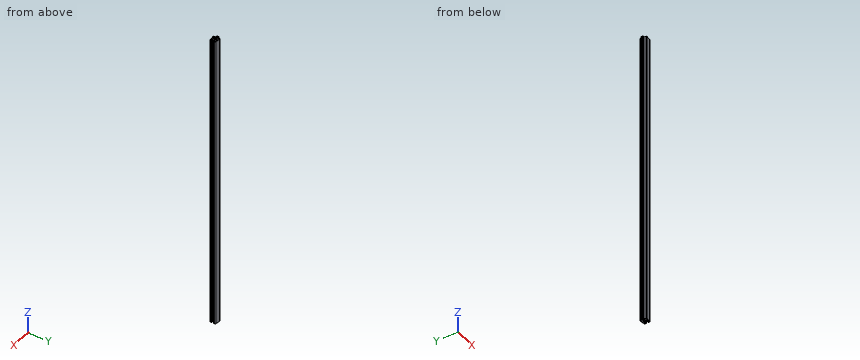
from build123d import *

# Parameters (mm, degrees)
EXTRUDE1_DEPTH = 1300


with BuildPart() as part:
    # Sketch1 → Extrude1 (new body)
    with BuildSketch(Plane.XY):
        with BuildLine():
            Line((21.490009074, 1.2), (22.34167412, 1.2))
            ThreePointArc((22.34167412, 1.2), (22.757184066, 1.325619119), (23.033504697, 1.66039604))
            ThreePointArc((23.033504697, 1.66039604), (23.959440841, 3.040559159), (25.33960396, 3.966495303))
            ThreePointArc((25.33960396, 3.966495303), (25.674380881, 4.242815934), (25.8, 4.65832588))
            Line((25.8, 4.65832588), (25.8, 5.509990926))
            ThreePointArc((25.8, 5.509990926), (25.846470105, 5.638164914), (25.964285714, 5.706776316))
            ThreePointArc((25.964285714, 5.706776316), (27, 5.8), (28.035714286, 5.706776316))
            ThreePointArc((28.035714286, 5.706776316), (28.153529895, 5.638164914), (28.2, 5.509990926))
            Line((28.2, 5.509990926), (28.2, 4.65832588))
            ThreePointArc((28.2, 4.65832588), (28.325619119, 4.242815934), (28.66039604, 3.966495303))
            ThreePointArc((28.66039604, 3.966495303), (30.040559159, 3.040559159), (30.966495303, 1.66039604))
            ThreePointArc((30.966495303, 1.66039604), (31.242815934, 1.325619119), (31.65832588, 1.2))
            Line((31.65832588, 1.2), (34.3, 1.2))
            Line((34.3, 1.2), (34.3, 5.944365081))
            ThreePointArc((34.3, 5.944365081), (34.315224093, 6.020901768), (34.358578644, 6.085786438))
            Line((34.358578644, 6.085786438), (39.053219906, 10.7804277))
            ThreePointArc((39.053219906, 10.7804277), (39.09082989, 10.804079854), (39.134973737, 10.809105395))
            Line((39.134973737, 10.809105395), (39.165647289, 10.805697223))
            ThreePointArc((39.165647289, 10.805697223), (40.117692027, 10.315253814), (40.5, 9.314871621))
            Line((40.5, 9.314871621), (40.5, 4.3))
            ThreePointArc((40.5, 4.3), (40.558578644, 4.158578644), (40.7, 4.1))
            Line((40.7, 4.1), (41.8, 4.1))
            ThreePointArc((41.8, 4.1), (41.941421356, 4.158578644), (42, 4.3))
            Line((42, 4.3), (42, 9.314871621))
            ThreePointArc((42, 9.314871621), (41.235384054, 11.315636008), (39.331294578, 12.296522825))
            Line((39.331294578, 12.296522825), (18.331294578, 14.629856158))
            ThreePointArc((18.331294578, 14.629856158), (15.999235613, 13.883589008), (15, 11.648204954))
            Line((15, 11.648204954), (15, 3.87298837))
            ThreePointArc((15, 3.87298837), (14.684748025, 3.408372219), (14.13652733, 3.529640706))
            ThreePointArc((14.13652733, 3.529640706), (13.848340865, 3.811685359), (13.538931751, 4.070271178))
            ThreePointArc((13.538931751, 4.070271178), (13.510259193, 4.105338584), (13.5, 4.149458734))
            Line((13.5, 4.149458734), (13.5, 5.04003891))
            ThreePointArc((13.5, 5.04003891), (13.470710678, 5.110749588), (13.4, 5.14003891))
            Line((13.4, 5.14003891), (10.4, 5.14003891))
            ThreePointArc((10.4, 5.14003891), (10.279875007, 5.138635031), (10.159815633, 5.134424161))
            ThreePointArc((10.159815633, 5.134424161), (8.129682846, 4.208865984), (7.3, 2.137701227))
            Line((7.3, 2.137701227), (7.3, 0.95))
            ThreePointArc((7.3, 0.95), (7.358578644, 0.808578644), (7.5, 0.75))
            Line((7.5, 0.75), (7.872649609, 0.75))
            ThreePointArc((7.872649609, 0.75), (7.986504617, 0.785570571), (8.059860749, 0.87962963))
            ThreePointArc((8.059860749, 0.87962963), (9.999819413, 2.467763258), (12.342238608, 1.574074074))
            ThreePointArc((12.342238608, 1.574074074), (12.4115514, 1.519465813), (12.497617696, 1.5))
            Line((12.497617696, 1.5), (13.5, 1.5))
            ThreePointArc((13.5, 1.5), (15, 0), (13.5, -1.5))
            Line((13.5, -1.5), (12.497617696, -1.5))
            ThreePointArc((12.497617696, -1.5), (12.4115514, -1.519465813), (12.342238608, -1.574074074))
            ThreePointArc((12.342238608, -1.574074074), (9.999819413, -2.467763258), (8.059860749, -0.87962963))
            ThreePointArc((8.059860749, -0.87962963), (7.986504617, -0.785570571), (7.872649609, -0.75))
            Line((7.872649609, -0.75), (7.5, -0.75))
            ThreePointArc((7.5, -0.75), (7.358578644, -0.808578644), (7.3, -0.95))
            Line((7.3, -0.95), (7.3, -2.137701227))
            ThreePointArc((7.3, -2.137701227), (8.129682846, -4.208865984), (10.159815633, -5.134424161))
            ThreePointArc((10.159815633, -5.134424161), (10.279875007, -5.138635031), (10.4, -5.14003891))
            Line((10.4, -5.14003891), (13.4, -5.14003891))
            ThreePointArc((13.4, -5.14003891), (13.470710678, -5.110749588), (13.5, -5.04003891))
            Line((13.5, -5.04003891), (13.5, -4.149458734))
            ThreePointArc((13.5, -4.149458734), (13.510259193, -4.105338584), (13.538931751, -4.070271178))
            ThreePointArc((13.538931751, -4.070271178), (13.848340865, -3.811685359), (14.13652733, -3.529640706))
            ThreePointArc((14.13652733, -3.529640706), (14.684748025, -3.408372219), (15, -3.87298837))
            Line((15, -3.87298837), (15, -11.648204954))
            ThreePointArc((15, -11.648204954), (15.999235613, -13.883589008), (18.331294578, -14.629856158))
            Line((18.331294578, -14.629856158), (39.331294578, -12.296522825))
            ThreePointArc((39.331294578, -12.296522825), (41.235384054, -11.315636008), (42, -9.314871621))
            Line((42, -9.314871621), (42, -4.3))
            ThreePointArc((42, -4.3), (41.941421356, -4.158578644), (41.8, -4.1))
            Line((41.8, -4.1), (40.7, -4.1))
            ThreePointArc((40.7, -4.1), (40.558578644, -4.158578644), (40.5, -4.3))
            Line((40.5, -4.3), (40.5, -9.314871621))
            ThreePointArc((40.5, -9.314871621), (40.117692027, -10.315253814), (39.165647289, -10.805697223))
            Line((39.165647289, -10.805697223), (39.134973737, -10.809105395))
            ThreePointArc((39.134973737, -10.809105395), (39.09082989, -10.804079854), (39.053219906, -10.7804277))
            Line((39.053219906, -10.7804277), (34.358578644, -6.085786438))
            ThreePointArc((34.358578644, -6.085786438), (34.315224093, -6.020901768), (34.3, -5.944365081))
            Line((34.3, -5.944365081), (34.3, -1.2))
            Line((34.3, -1.2), (31.65832588, -1.2))
            ThreePointArc((31.65832588, -1.2), (31.242815934, -1.325619119), (30.966495303, -1.66039604))
            ThreePointArc((30.966495303, -1.66039604), (30.040559159, -3.040559159), (28.66039604, -3.966495303))
            ThreePointArc((28.66039604, -3.966495303), (28.325619119, -4.242815934), (28.2, -4.65832588))
            Line((28.2, -4.65832588), (28.2, -5.509990926))
            ThreePointArc((28.2, -5.509990926), (28.153529895, -5.638164914), (28.035714286, -5.706776316))
            ThreePointArc((28.035714286, -5.706776316), (27, -5.8), (25.964285714, -5.706776316))
            ThreePointArc((25.964285714, -5.706776316), (25.846470105, -5.638164914), (25.8, -5.509990926))
            Line((25.8, -5.509990926), (25.8, -4.65832588))
            ThreePointArc((25.8, -4.65832588), (25.674380881, -4.242815934), (25.33960396, -3.966495303))
            ThreePointArc((25.33960396, -3.966495303), (23.959440841, -3.040559159), (23.033504697, -1.66039604))
            ThreePointArc((23.033504697, -1.66039604), (22.757184066, -1.325619119), (22.34167412, -1.2))
            Line((22.34167412, -1.2), (21.490009074, -1.2))
            ThreePointArc((21.490009074, -1.2), (21.361835086, -1.153529895), (21.293223684, -1.035714286))
            ThreePointArc((21.293223684, -1.035714286), (21.2, 0), (21.293223684, 1.035714286))
            ThreePointArc((21.293223684, 1.035714286), (21.361835086, 1.153529895), (21.490009074, 1.2))
        make_face()
        with BuildLine():
            Line((16.5, -1.25), (16.5, -11.648204954))
            ThreePointArc((16.5, -11.648204954), (16.999617806, -12.765896981), (18.165647289, -13.139030556))
            Line((18.165647289, -13.139030556), (36.764437067, -11.072498358))
            ThreePointArc((36.764437067, -11.072498358), (36.931076425, -10.939923), (36.883772118, -10.732300255))
            Line((36.883772118, -10.732300255), (33.510050506, -7.358578644))
            ThreePointArc((33.510050506, -7.358578644), (33.445165837, -7.315224093), (33.36862915, -7.3))
            Line((33.36862915, -7.3), (27, -7.3))
            ThreePointArc((27, -7.3), (22.343811305, -5.622268833), (19.827850799, -1.360248447))
            ThreePointArc((19.827850799, -1.360248447), (19.569361706, -0.92236964), (19.090986155, -0.75))
            Line((19.090986155, -0.75), (17, -0.75))
            ThreePointArc((17, -0.75), (16.646446609, -0.896446609), (16.5, -1.25))
        make_face(mode=Mode.SUBTRACT)
        with BuildLine():
            Line((17, 0.75), (19.090986155, 0.75))
            ThreePointArc((19.090986155, 0.75), (19.569361706, 0.92236964), (19.827850799, 1.360248447))
            ThreePointArc((19.827850799, 1.360248447), (22.343811305, 5.622268833), (27, 7.3))
            Line((27, 7.3), (33.36862915, 7.3))
            ThreePointArc((33.36862915, 7.3), (33.445165837, 7.315224093), (33.510050506, 7.358578644))
            Line((33.510050506, 7.358578644), (36.883772118, 10.732300255))
            ThreePointArc((36.883772118, 10.732300255), (36.931076425, 10.939923), (36.764437067, 11.072498358))
            Line((36.764437067, 11.072498358), (18.165647289, 13.139030556))
            ThreePointArc((18.165647289, 13.139030556), (16.999617806, 12.765896981), (16.5, 11.648204954))
            Line((16.5, 11.648204954), (16.5, 1.25))
            ThreePointArc((16.5, 1.25), (16.646446609, 0.896446609), (17, 0.75))
        make_face(mode=Mode.SUBTRACT)
    extrude(amount=EXTRUDE1_DEPTH)


solid = part.part
For this review, take the finished solid that the model builds, in its own axes (mm). Give positions to 0.01 mm unless a question says otherwise; leave off trailing zeros.
Item 1: Insertion check: pin 1 (0.7 mm diameter, centred on y = -5, z = 495, fed in from -X); pin 2 (10 mm diameter, centred on x = 25, z = 509.5, fed in from +Y); pin 3 (1.3 mm diameter, centred on x = 32.5, z = 567, fed in from +Y). Each pin has a flat end and moves straight along its axis. Give the tip position at first contact, or say it passes through.
Item 2: For line 1 along X through (y, z) = (8.25, 171); line 2 along Y through (x, z) = (30.5, 472.5); line 3 along X through (y, z) = (-2.25, 90.5), list the stretches that pass through material, from the lowest coordinate up.
Item 3: Take a section at A-A, the plane z = 772.5. Give the number of separate pieces and of enclosed holes in the cut face, and give its area (3 significant figures).
Calculated:
1. pin 1: stops at x = 8.66
1. pin 2: stops at y = 14.44
1. pin 3: stops at y = 13.13
2. line 1: x = 15 to 16.5, 34.4 to 36.52, 40.5 to 42
2. line 2: y = -13.28 to -11.77, -7.3 to -2.5, 2.5 to 7.3, 11.77 to 13.28
2. line 3: x = 7.3 to 9.31, 11.49 to 16.5, 20.06 to 23.34, 30.66 to 34.3
3. separate pieces: 1
3. enclosed holes: 2
3. area: 315 mm2
